```python
from build123d import *

# Parameters (mm, degrees)
BOSS_EXTRUDE1_DEPTH = 2
FILLET2_R           = 0.5
SKETCH2_R           = 5.5
CUT_EXTRUDE1_DEPTH  = 3.0000001
SCALE1_SCALE        = 0.05848


with BuildPart() as part:
    # Sketch1 → Boss-Extrude1 (new body)
    with BuildSketch(Plane(origin=(0, 0, 0), x_dir=(1, 0, 0), z_dir=(0, 1, 0))):
        with BuildLine():
            Line((92.085110733, 127.103938413), (77.178124527, 138.062250462))
            Line((77.178124527, 138.062250462), (70.360301054, 128.787719859))
            Line((70.360301054, 128.787719859), (80.370912811, 121.428793922))
            Line((80.370912811, 121.428793922), (45.876712151, 73.307436464))
            add(Edge.make_bspline(
                [(33.451049577, 53.126345945), (31.215883749, 60.494948343), (32.447141404, 70.446648696), (40.862115825, 73.16760251), (45.876712151, 73.307436464)],
                knots=[0, 0, 0, 0, 0.641849019, 1, 1, 1, 1], degree=3))
            Line((33.451049577, 53.126345945), (-106.799876202, -136.181201423))
            ThreePointArc((-106.799876202, -136.181201423), (-106.088492795, -137.707043736), (-104.423962902, -137.959236822))
            Line((-104.423962902, -137.959236822), (37.646178322, 49.986884833))
            add(Edge.make_bspline(
                [(37.646178322, 49.986884833), (45.3460396, 49.920523216), (54.546555656, 53.908359677), (54.783891194, 62.749120731), (53.503843784, 67.599606116)],
                knots=[0, 0, 0, 0, 0.641849019, 1, 1, 1, 1], degree=3))
            Line((53.503843784, 67.599606116), (89.943937285, 114.264737729))
            Line((89.943937285, 114.264737729), (99.827328979, 106.735813017))
            Line((99.827328979, 106.735813017), (106.802651201, 115.89247806))
            Line((106.802651201, 115.89247806), (92.085110733, 127.103938413))
        make_face()
    extrude(amount=BOSS_EXTRUDE1_DEPTH)

    # Fillet2
    fillet2_edges = [part.edges().sort_by_distance(p)[0] for p in [
        (-104.423962902, 1, 137.959236822),
        (-106.799876202, 1, 136.181201423),
        (33.451049577, 1, -53.126345945),
        (37.646178322, 1, -49.986884833),
        (45.876712151, 1, -73.307436464),
        (53.503843784, 1, -67.599606116),
        (99.827328979, 1, -106.735813017),
        (89.943937285, 1, -114.264737729),
        (80.370912811, 1, -121.428793922),
        (70.360301054, 1, -128.787719859),
        (77.178124527, 1, -138.062250462),
        (106.802651201, 1, -115.89247806),
    ]]
    fillet(fillet2_edges, radius=FILLET2_R)

    # Sketch2 → Cut-Extrude1 (cut, through all)
    with BuildSketch(Plane(origin=(0, 2, 0), x_dir=(1, 0, 0), z_dir=(0, 1, 0))):
        with Locations((43.025259326, 61.547339532)):
            Circle(SKETCH2_R)
    extrude(amount=-CUT_EXTRUDE1_DEPTH, mode=Mode.SUBTRACT)


with BuildPart() as part_1:
    # Scale1: scaled about (28.469603302, 1, -42.097394776)
    add(part.part.scale(SCALE1_SCALE).moved(Location((26.804700901, 0.94152, -39.635539129))))


solid = part_1.part
```
For this review, take the finished solid that the model builds, in its own axes (mm). Coordinates: 2 decimals unless noted, no trailing zeros. Order: outer loops, then holes, each group sorted by start corner. A loop starts at its lowest first (then second) coordinate and runs counter-clockwise, first axis right, second up. Notation, with made-up numbers: (-35.5, -5) - (-22.5, -5) arc R25 ccw to (-22.5, 18) - close; hole circle Ø5 at (-23, 49.25). An arc over 180 degrees is marked (long way). Answer as a JSON object with one key per item and string values. Group by question number.
1. For probe 1 along Z at (x, y) = (31, 1); probe 2 along Z at (x, y) = (22.5, 1); probe 3 along X at (y, z) = (1, -32.5), list the stretches that pass through material, from the lowest coordinate up.
2. We need section A-A on z = -39. State the section outline as (x, y) points, then the cut area to 3 significant figures.
3. We need section B-B on x = 22.5. State the section outline as (y, z) points, then the cut area to 3 significant figures.
Final values:
{
 "1": {"probe 1": "-47.28 to -47.11, -46.03 to -44.95", "probe 2": "-34.29 to -33.95", "probe 3": "21.17 to 21.4"},
 "2": {"outline": "(25.99, 0.94) - (26.32, 0.94) - (26.32, 1.06) - (25.99, 1.06) - close", "area": "0.0383 mm²"},
 "3": {"outline": "(0.94, -34.29) - (1.06, -34.29) - (1.06, -33.95) - (0.94, -33.95) - close", "area": "0.0398 mm²"}
}
